from build123d import *

# Parameters (mm, degrees)
IZIM3_W                                          = 3.5
IZIM3_H                                          = 23
IZIM3_H_2                                        = 5
IZIM3_W_2                                        = 2.5
Y_KSEKLIK_EKSTR_ZYON3_DEPTH                      = 8.28
IZIM4_W                                          = 7
IZIM4_H                                          = 5.16
KES_EKSTR_ZYON1_DEPTH                            = 34
IZIM11_W                                         = 12
IZIM11_H                                         = 33
KES_EKSTR_ZYON2_DEPTH                            = 1
M2_D_Z_BA_L_MAKINE_VIDAS_IN_HAV_A_DE_D           = 2
M2_D_Z_BA_L_MAKINE_VIDAS_IN_HAV_A_DE_CSINK_D     = 2.6
M2_D_Z_BA_L_MAKINE_VIDAS_IN_HAV_A_DE_CSINK_ANGLE = 90


with BuildPart() as part:
    # Çizim3 → Yükseklik-Ekstrüzyon3 (new body)
    with BuildSketch(Plane(origin=(0, 0, 0), x_dir=(1, 0, 0), z_dir=(0, 1, 0))):
        with BuildLine():
            Line((16, 6.5), (16, 11.5))
            Line((16, 11.5), (11.324751653, 11.5))
            ThreePointArc((11.324751653, 11.5), (10.819882158, 9.603828792), (10, 7.821091654))
            Line((10, 7.821091654), (10, -21.5))
            Line((10, -21.5), (16, -21.5))
            Line((16, -21.5), (16, -16.5))
            Line((16, -16.5), (16, 6.5))
        make_face()
        with Locations((17.75, -5)):
            Rectangle(IZIM3_W, IZIM3_H)
        with Locations((17.75, 9)):
            Rectangle(IZIM3_W, IZIM3_H_2)
        with Locations((20.75, 9)):
            Rectangle(IZIM3_W_2, IZIM3_H_2)
        with Locations((17.75, -19)):
            Rectangle(IZIM3_W, IZIM3_H_2)
        with Locations((20.75, -19)):
            Rectangle(IZIM3_W_2, IZIM3_H_2)
    extrude(amount=Y_KSEKLIK_EKSTR_ZYON3_DEPTH)

    # Çizim4 → Kes-Ekstrüzyon1 (cut, through all)
    with BuildSketch(Plane.XY.offset(21.5)):
        with Locations((13.5, 2.58)):
            Rectangle(IZIM4_W, IZIM4_H)
    extrude(amount=-KES_EKSTR_ZYON1_DEPTH, mode=Mode.SUBTRACT)

    # Çizim11 → Kes-Ekstrüzyon2 (cut)
    with BuildSketch(Plane(origin=(0, 8.28, 0), x_dir=(1, 0, 0), z_dir=(0, 1, 0))):
        with Locations((16, -5)):
            Rectangle(IZIM11_W, IZIM11_H)
    extrude(amount=-KES_EKSTR_ZYON2_DEPTH, mode=Mode.SUBTRACT)

    # M2 Düz Başlı Makine Vidası İçin Havşa_ DEĞİŞTİREBİLİRİZ (through all)
    with Locations(Plane(origin=(19.5, 7.28, 19), x_dir=(0, 0, 1), z_dir=(0, 1, 0))):
        with Locations((0, 0), (-28, 0), (-2, -6), (-10, -6), (-18, -6), (-26, -6)):
            CounterSinkHole(M2_D_Z_BA_L_MAKINE_VIDAS_IN_HAV_A_DE_D / 2, M2_D_Z_BA_L_MAKINE_VIDAS_IN_HAV_A_DE_CSINK_D / 2, counter_sink_angle=M2_D_Z_BA_L_MAKINE_VIDAS_IN_HAV_A_DE_CSINK_ANGLE)


solid = part.part
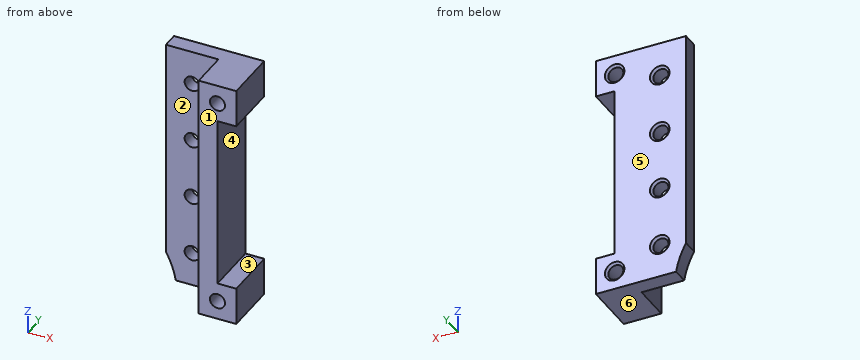
Work out the finished part from the listing and answer in its coordinate system (mm). Face numbers are marked on the shaded views. A direction names the side the tool comes from. Coordinates: 2 decimals unless noted, no trailing zeros. Order: outer loops, then holes, each group sorted by start corner. A loop starts at its lowest first (then second) coordinate and runs counter-clockwise, first axis right, second up. Notation, with made-up numbers: (88.25, 6.25) - (94.25, 6.25) arc R29 cw to (94.25, 30.25) - close; hole circle Ø11 at (38.5, 25.25). An arc over 180 degrees is marked (long way). Put each result on its own line as item: value. Start each with the question number.
1) Find section C-C (z = -4.5). Give the vertices of the cut face in (x, y), plus the area to 3 significant figures.
2) Find section D-D (x = 19). State how many separate pieces and enclosed holes the cut face has, plus the area to 3 significant figures.
3) For a pull along Z with two mould halves and no side action, classify the marked faces 4, 5 and 6 as released by +Z, released by -Z, zero draft, split by the parting line, or undercut.
4) For the marked faces 1, 2 and 3, determine the directions among +Z, -Z, +X, -X, +Y, -Y from which every point of the face is accessible in a straight line to the end or side of a thin tool.
5) Find section A-A (z = 9). Give the vertices of the cut face in (x, y).
6) Flat-ended cylindrical pins translate along their axes: pin 1 (1.6 mm diameter, centred on x = 13.5, z = 1, fed in from -Y); pin 2 (3 mm diameter, centred on y = 2.5, z = -1, fed in from +X); pin 3 (1.5 mm diameter, centred on y = 2.5, z = -7, fed in from -X); pin 4 (3 mm diameter, centred on x = 12, y = 4, fed in from -Z). Find the tip coordinate at first contact, or state that the pin passes through.
7) Find the intervals of material crossed by line 1 (Z direction, x = 13.5, y = 5.65); line 2 (X direction, y = 5, z = -9); line 3 (X direction, y = 6.25, z = 1), in increasing order. Write a range as from..to.
8) Find section B-B (y = 1.75). Give the vertices of the cut face in (x, z), plus the area to 3 significant figures.
Results list:
1. outline: (10, 5.16) - (17, 5.16) - (17, 0) - (19.5, 0) - (19.5, 7.28) - (10, 7.28) - close
1. area: 33.0 mm^2
2. separate pieces: 3
2. enclosed holes: 0
2. area: 215 mm^2
3. face 4: undercut
3. face 5: zero draft
3. face 6: released by -Z
4. face 1: +Z, -Z, +X, -X, -Y
4. face 2: +Z, -Z, -X, -Y
4. face 3: +X, +Y, -Y
5. outline: (10, 5.16) - (12.5, 5.16) - (12.5, 6.98) - (12.2, 7.28) - (10, 7.28) - close; (14.5, 5.16) - (17, 5.16) - (17, 0) - (19.5, 0) - (19.5, 7.28) - (14.8, 7.28) - (14.5, 6.98) - close
6. pin 1: passes through
6. pin 2: stops at x = 19.5
6. pin 3: stops at x = 17
6. pin 4: stops at z = -11.5
7. line 1: z = -11.5..-8, -6..0, 2..8, 10..16, 18..21.5
7. line 2: x = 17..18.5, 20.5..22
7. line 3: x = 10..12.5, 14.5..19.5
8. outline: (17, -11.5) - (22, -11.5) - (22, -6.5) - (19.5, -6.5) - (19.5, 16.5) - (22, 16.5) - (22, 21.5) - (17, 21.5) - close; hole circle Ø2 at (19.5, -9); hole circle Ø2 at (19.5, 19)
8. area: 101 mm^2
